Here's how the part is built. I have some questions about the finished solid (model axes, mm). Face numbers are marked on the shaded views. A direction names the side the tool comes from. Coordinates: 2 decimals unless noted, no trailing zeros. Write each loop counter-clockwise with the first axis right and the second up, starting at its lowest first coordinate (ties: lowest second). Pieces come first, ordered by that corner, then holes. Notation, with made-up numbers: (64, 13.5) -> (69, 13.5) arc R12 ccw to (69, 29.5) -> close; hole circle Ø6 at (58.25, 55.5). An arc over 180 degrees is marked (long way). Answer in a Markdown table with one row per item. Add a question column.
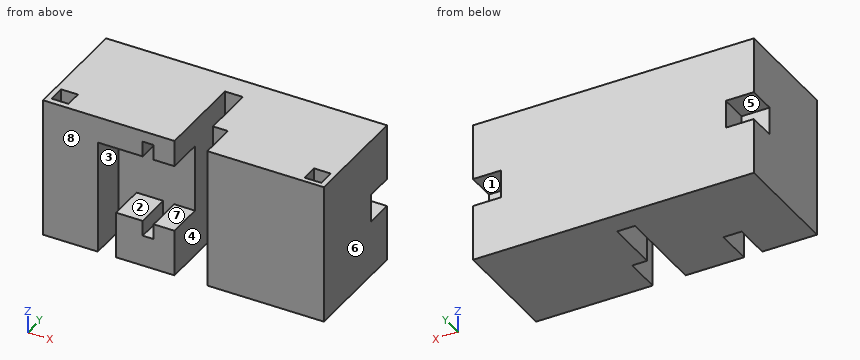
from build123d import *

# Parameters (mm, degrees)
SKETCH1_W                = 100
SKETCH1_H                = 100
BOSS_EXTRUDE1_DEPTH      = 50
BOSS_EXTRUDE4_DEPTH      = 50
BOSS_EXTRUDE4_2_DEPTH    = 50
SKETCH11_W               = 100
SKETCH11_H               = 50
CUT_EXTRUDE4_DEPTH       = 100
SKETCH13_W               = 100
SKETCH13_H               = 10
CUT_EXTRUDE5_DEPTH       = 50
SKETCH2_W                = 50
SKETCH2_H                = 50
CUT_EXTRUDE6_DEPTH       = 25
BOSS_EXTRUDE5_DEPTH      = 19.5
CUT_EXTRUDE7_DEPTH       = 12
CUT_EXTRUDE8_DEPTH       = 32
SKETCH27_W               = 6.4
SKETCH27_H               = 32
CUT_EXTRUDE9_DEPTH       = 29
SKETCH29_W               = 6
SKETCH29_H               = 3.5
CUT_EXTRUDE10_DEPTH      = 28
SKETCH30_W               = 100
SKETCH30_H               = 50
CUT_EXTRUDE11_DEPTH      = 45
SKETCH32_W               = 9.8
SKETCH32_H               = 9.8
BOSS_EXTRUDE6_DEPTH      = 9.8
CHAMFER1_SIZE            = 1
BOSS_EXTRUDE7_DEPTH      = 13
SKETCH34_3_W             = 9.7
SKETCH34_3_H             = 8.5
SKETCH34_3_W_2           = 0.5
SKETCH34_3_H_2           = 13.5
SKETCH34_3_H_3           = 16.6
SKETCH34_3_W_3           = 6
CUT_EXTRUDE12_DEPTH      = 13
CUT_EXTRUDE13_DEPTH      = 82.240384046
CUT_EXTRUDE13_DEPTH_BACK = 10
SKETCH36_W               = 10
SKETCH36_H               = 10
SKETCH37_W               = 9.8
SKETCH37_H               = 9.8
SKETCH37_H_2             = 10.048829857
CUT_EXTRUDE15_DEPTH      = 10
SKETCH38_W               = 6
SKETCH38_H               = 6
CUT_EXTRUDE16_DEPTH      = 6
SKETCH39_W               = 6.4
SKETCH39_H               = 16.6
CUT_EXTRUDE17_DEPTH      = 32
CUT_EXTRUDE18_DEPTH      = 13


with BuildPart() as part:
    # Sketch1 → Boss-Extrude1 (new body)
    with BuildSketch(Plane(origin=(0, 0, 0), x_dir=(1, 0, 0), z_dir=(0, 1, 0))):
        Rectangle(SKETCH1_W, SKETCH1_H)
    extrude(amount=-BOSS_EXTRUDE1_DEPTH)

    # Sketch13 → Cut-Extrude5 (cut)
    with BuildSketch(Plane(origin=(0, 0, -50), x_dir=(-1, 0, 0), z_dir=(0, 0, -1))):
        with Locations((0, -45)):
            Rectangle(SKETCH13_W, SKETCH13_H)
    extrude(amount=-CUT_EXTRUDE5_DEPTH, mode=Mode.SUBTRACT)

    # Sketch2 → Cut-Extrude6 (cut)
    with BuildSketch(Plane(origin=(0, 0, 0), x_dir=(1, 0, 0), z_dir=(0, 1, 0))):
        with Locations((-25, -25)):
            Rectangle(SKETCH2_W, SKETCH2_H)
        with Locations((25, -25)):
            Rectangle(SKETCH2_W, SKETCH2_H)
    extrude(amount=-CUT_EXTRUDE6_DEPTH, mode=Mode.SUBTRACT)

    # Sketch18 → Boss-Extrude5 (add)
    with BuildSketch(Plane(origin=(0, 0, 0), x_dir=(-1, 0, 0), z_dir=(0, 0, -1))):
        Polygon((50, -50), (50, -70), (30, -50), align=None)
        Polygon((-50, -50), (-50, -69.5), (-30.5, -50), align=None)
    extrude(amount=-BOSS_EXTRUDE5_DEPTH)

    # Sketch20 → Cut-Extrude7 (cut)
    with BuildSketch(Plane.XZ.offset(40)):
        Polygon((3.2, 0), (0, 0), (-30, 0), (-30, -22.9), (-14, -22.9), (-14, -27.9), (-11.1, -27.9), (-11.1, -22.9), (-7, -22.9), (-7, -14.9), (-2.8, -14.9), (3.2, -14.9), align=None)
    extrude(amount=-CUT_EXTRUDE7_DEPTH, mode=Mode.SUBTRACT)

    # Sketch21 → Cut-Extrude8 (cut)
    with BuildSketch(Plane.XZ.offset(40)):
        Polygon((3.2, 0), (0, 0), (-3.2, 0), (-3.2, -14.9), (3.2, -14.9), align=None)
    extrude(amount=-CUT_EXTRUDE8_DEPTH, mode=Mode.SUBTRACT)

    # Sketch27 → Cut-Extrude9 (cut)
    with BuildSketch(Plane(origin=(0, 0, 0), x_dir=(-1, 0, 0), z_dir=(0, 0, -1))):
        with Locations((0, -34)):
            Rectangle(SKETCH27_W, SKETCH27_H)
    extrude(amount=-CUT_EXTRUDE9_DEPTH, mode=Mode.SUBTRACT)

    # Sketch29 → Cut-Extrude10 (cut)
    with BuildSketch(Plane(origin=(0, 0, -50), x_dir=(-1, 0, 0), z_dir=(0, 0, -1))):
        Polygon((24, -34), (24, -36.5), (30, -36.5), (30, -31.5), (24, -31.5), align=None)
        with Locations((27, -38.25)):
            Rectangle(SKETCH29_W, SKETCH29_H)
    extrude(amount=-CUT_EXTRUDE10_DEPTH, mode=Mode.SUBTRACT)

    # Sketch30 → Cut-Extrude11 (cut)
    with BuildSketch(Plane(origin=(0, -25, 0), x_dir=(1, 0, 0), z_dir=(0, 1, 0))):
        with Locations((0, -25)):
            Rectangle(SKETCH30_W, SKETCH30_H)
    extrude(amount=-CUT_EXTRUDE11_DEPTH, mode=Mode.SUBTRACT)

    # Sketch32 → Boss-Extrude6 (add)
    with BuildSketch(Plane.XY):
        with Locations((-45.1, -35.1)):
            Rectangle(SKETCH32_W, SKETCH32_H)
        with Locations((45.1, -35.1)):
            Rectangle(SKETCH32_W, SKETCH32_H)
    extrude(amount=BOSS_EXTRUDE6_DEPTH)

    # Chamfer1
    chamfer1_edges = [part.edges().sort_by_distance(p)[0] for p in [
        (-40.2, -40, 4.9),
        (-40.2, -30.2, 4.9),
        (-40.2, -35.1, 9.8),
        (40.2, -30.2, 4.9),
        (40.2, -35.1, 9.8),
    ]]
    chamfer(chamfer1_edges, length=CHAMFER1_SIZE)

    # Sketch34 → Boss-Extrude7 (add)
    with BuildSketch(Plane.XZ.offset(40)):
        Polygon((-30, 0), (-30, -9.4), (-14.5, -9.4), (-14.5, -3.9), (-10.6, -3.9), (-10.6, -9.4), (-3.2, -9.4), (-3.2, 0), align=None)
    extrude(amount=-BOSS_EXTRUDE7_DEPTH)

    # Sketch34<3> → Cut-Extrude12 (cut)
    with BuildSketch(Plane.XZ.offset(40)):
        Polygon((3.2, -9.4), (3.2, -14.9), (3.2, -24.9), (8.5, -24.9), (8.5, 0), (3.2, 0), align=None)
        Polygon((-14, -27.9), (-11.1, -27.9), (-11.1, -22.9), (-7, -22.9), (-7, -14.9), (3.2, -14.9), (3.2, -9.4), (-3.2, -9.4), (-10.6, -9.4), (-10.6, -3.9), (-14.5, -3.9), (-14.5, -9.4), (-30, -9.4), (-30, -22.9), (-24, -22.9), (-14, -22.9), align=None)
        Polygon((-11.1, -22.9), (-11.1, -27.9), (-14, -27.9), (-14, -22.9), (-24, -22.9), (-24, -33.4), (-14.5, -33.4), (-14.5, -38.9), (-10.6, -38.9), (-10.6, -33.4), (-6.5, -33.4), (-6.5, -24.9), (3.2, -24.9), (3.2, -14.9), (-7, -14.9), (-7, -22.9), align=None)
        with Locations((-1.65, -29.15)):
            Rectangle(SKETCH34_3_W, SKETCH34_3_H)
        Polygon((-24, -33.4), (-24, -22.9), (-30, -22.9), (-30.5, -22.9), (-30.5, -33.4), (-30, -33.4), align=None)
        with Locations((-30.25, -16.15)):
            Rectangle(SKETCH34_3_W_2, SKETCH34_3_H_2)
        with Locations((-30.25, -41.7)):
            Rectangle(SKETCH34_3_W_2, SKETCH34_3_H_3)
        with Locations((-27, -41.7)):
            Rectangle(SKETCH34_3_W_3, SKETCH34_3_H_3)
    extrude(amount=-CUT_EXTRUDE12_DEPTH, mode=Mode.SUBTRACT)

    # Sketch36 → Cut-Extrude13 (cut, two sides: drawn at the far end of the back side and taken through both)
    with BuildSketch(Plane(origin=(0, 0, 0), x_dir=(1, 0, 0), z_dir=(0, 1, 0)).offset(-CUT_EXTRUDE13_DEPTH_BACK)):
        with Locations((-45, 25)):
            Rectangle(SKETCH36_W, SKETCH36_H)
        Polygon((50, 20), (50, 30), (40, 30), (40, 25), (40, 20), align=None)
    extrude(amount=CUT_EXTRUDE13_DEPTH + CUT_EXTRUDE13_DEPTH_BACK, mode=Mode.SUBTRACT)

    # Sketch37 → Cut-Extrude15 (cut)
    with BuildSketch(Plane.XZ.offset(40)):
        with Locations((-45.1, 4.9)):
            Rectangle(SKETCH37_W, SKETCH37_H)
        with Locations((45.1, 5.024414929)):
            Rectangle(SKETCH37_W, SKETCH37_H_2)
    extrude(amount=-CUT_EXTRUDE15_DEPTH, mode=Mode.SUBTRACT)

    # Sketch38 → Cut-Extrude16 (cut)
    with BuildSketch(Plane.XY):
        with Locations((-45.1, -34.890503426)):
            Rectangle(SKETCH38_W, SKETCH38_H)
        with Locations((45.1, -35.230904897)):
            Rectangle(SKETCH38_W, SKETCH38_H)
    extrude(amount=-CUT_EXTRUDE16_DEPTH, mode=Mode.SUBTRACT)

    # Sketch39 → Cut-Extrude17 (cut)
    with BuildSketch(Plane.XZ.offset(40)):
        with Locations((0, -41.7)):
            Rectangle(SKETCH39_W, SKETCH39_H)
        Polygon((3.2, -14.9), (-3.2, -14.9), (-3.2, -33.4), (3.2, -33.4), (3.2, -24.9), align=None)
    extrude(amount=-CUT_EXTRUDE17_DEPTH, mode=Mode.SUBTRACT)

    # Sketch34<4> → Cut-Extrude18 (cut)
    with BuildSketch(Plane.XZ.offset(40)):
        Polygon((8.5, -24.9), (3.2, -24.9), (3.2, -33.4), (3.2, -50), (8.5, -50), align=None)
    extrude(amount=-CUT_EXTRUDE18_DEPTH, mode=Mode.SUBTRACT)


with BuildPart() as body_2:
    # Sketch6 → Boss-Extrude4 (new body)
    with BuildSketch(Plane.XY.offset(50)):
        with BuildLine():
            Line((-1.9e-08, -50), (-50, -50))
            Line((-50, -50), (-50, -63.397459622))
            ThreePointArc((-50, -63.397459622), (-25.88190452, -53.407417374), (-1.9e-08, -50))
        make_face()
    extrude(amount=-BOSS_EXTRUDE4_DEPTH)


with BuildPart() as body_3:
    # Sketch6 → Boss-Extrude4 2 (new body)
    with BuildSketch(Plane.XY.offset(50)):
        with BuildLine():
            Line((50, -50), (-1.9e-08, -50))
            ThreePointArc((-1.9e-08, -50), (25.881904501, -53.407417369), (50, -63.397459622))
            Line((50, -63.397459622), (50, -50))
        make_face()
    extrude(amount=-BOSS_EXTRUDE4_2_DEPTH)


with BuildPart() as cut_extrude4_tool:
    # Sketch11 → Cut-Extrude4 (new body)
    with BuildSketch(Plane(origin=(0, -63.397459622, 0), x_dir=(-1, 0, 0), z_dir=(0, -1, 0))):
        with Locations((0, -25)):
            Rectangle(SKETCH11_W, SKETCH11_H)
    extrude(amount=-CUT_EXTRUDE4_DEPTH)


with BuildPart() as body_2_1:
    add(body_2.part)

    # Cut-Extrude4: cut by cut_extrude4_tool
    add(cut_extrude4_tool.part, mode=Mode.SUBTRACT)


with BuildPart() as body_3_1:
    add(body_3.part)

    # Cut-Extrude4: cut by cut_extrude4_tool
    add(cut_extrude4_tool.part, mode=Mode.SUBTRACT)


solid = part.part
Q1. For the marked faces 1, 2, 3, 4 and 5, which set-ups out of +Z, -Z, +X, -X, +Y, -Y let a thin tool reach every point of the face, with its end or its side?
Q2. Imagine slicing it at D-D on z = -26. Please give me the cut outline in (x, y), plus the area to 3 significant figures.
Q3. Imagine slicing it at A-A on y = -36.5. State how many separate pieces and enclosed holes the cut face has, plus the area to 3 significant figures.
Q4. Imagine slicing it at B-B on z = -5. Please give me the cut outline in (x, y), plus the area to 3 significant figures.
Q5. I'm going to push flat-ended pins straight in: P1, Ø8, axis at x = -15, z = -21, coming from the -Y side; P2, Ø5, axis at x = 45, z = -25, coming from the +Y side. Where does each tip first touch, or does it pass through?
Q6. If we mould it in two halves opening along X, with no side actions, what happens to the marked faces 6, 7 and 8? For each: pulls with the +X half, pulls with the -X half, needs draft (parallel to the pull), parting line crosses it, or undercut.
Q7. I need wall thicknesses on line 1 (X direction, y = -36.5, z = -36); line 2 (X direction, y = -15, z = -21.5); line 3 (Z direction, x = -5.5, y = -38). Which ranges of each line are inside material? Lowest first, please. Write a range as [from, to].
Q8. Imagine slicing it at C-C on y = -25. Please give me the cut outline in (x, z).
Result sheet:
| question | item | result |
|---|---|---|
| 1 | face 1 | +X, +Y |
| 1 | face 2 | -Y |
| 1 | face 3 | -Z, -Y |
| 1 | face 4 | +Z, -Z, -Y |
| 1 | face 5 | -X, +Y |
| 2 | outline | (-50, -40) -> (-30.5, -40) -> (-30.5, -27) -> (-3.2, -27) -> (-3.2, -8) -> (3.2, -8) -> (3.2, -27) -> (8.5, -27) -> (8.5, -40) -> (50, -40) -> (50, -10) -> (40, -10) -> (40, 0) -> (-40, 0) -> (-40, -10) -> (-50, -10) -> close |
| 2 | area | 3,170 mm^2 |
| 3 | separate pieces | 3 |
| 3 | enclosed holes | 0 |
| 3 | area | 3,540 mm^2 |
| 4 | outline | (-50, -40) -> (-14.5, -40) -> (-14.5, -27) -> (-10.6, -27) -> (-10.6, -40) -> (-3.2, -40) -> (-3.2, -8) -> (3.2, -8) -> (3.2, -27) -> (8.5, -27) -> (8.5, -40) -> (50, -40) -> (50, 0) -> (-50, 0) -> close; hole (-48.1, -37.89) -> (-42.1, -37.89) -> (-42.1, -31.89) -> (-48.1, -31.89) -> close; hole (42.1, -38.23) -> (48.1, -38.23) -> (48.1, -32.23) -> (42.1, -32.23) -> close |
| 4 | area | 3,600 mm^2 |
| 5 | P1 | stops at y = -27 |
| 5 | P2 | stops at y = -10 |
| 6 | face 6 | pulls with the +X half |
| 6 | face 7 | undercut |
| 6 | face 8 | needs draft |
| 7 | line 1 | x = [-50, -30.5], [-24, -14.5], [-10.6, -3.2], [8.5, 50] |
| 7 | line 2 | x = [-50, -3.2], [3.2, 50] |
| 7 | line 3 | z = [-50, -33.4], [-9.4, 0] |
| 8 | outline | (-50, -50) -> (-3.2, -50) -> (-3.2, 0) -> (-50, 0) -> close; (3.2, -50) -> (50, -50) -> (50, 0) -> (3.2, 0) -> close |
